```python
from build123d import *

# Parameters (mm, degrees)
F0_W     = 180
F0_H     = 150
F1_DEPTH = 20
F2_W     = 10
F2_H     = 150
F3_DEPTH = 20


# Not quite as in the source:
# - the program builds the solid bodies; features that only make, move or delete a surface that nothing else refers to are left out


with BuildPart() as f1:
    # F0 (on Right) → F1 (new body)
    with BuildSketch(Plane.YZ):
        with Locations((6.5838837624, 31.891247511)):
            Rectangle(F0_W, F0_H)
    extrude(amount=F1_DEPTH)

    # F2 (on face) → F3 (cut)
    with BuildSketch(Plane.XZ.offset(83.4161162376)):
        with Locations((15, 31.891247511)):
            Rectangle(F2_W, F2_H)
    extrude(amount=-F3_DEPTH, mode=Mode.SUBTRACT)


solid = f1.part
```
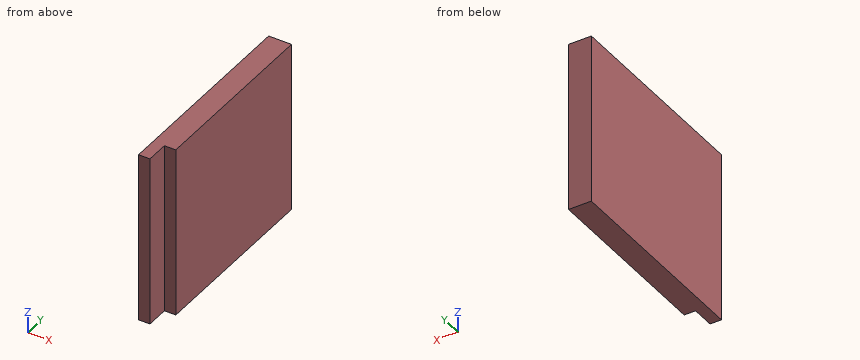
Geometry check sheet. Reference: the model listing, model coordinates, mm. Coordinates: 2 decimals unless noted, no trailing zeros. Loops run counter-clockwise (first coordinate to the right, second up) from the corner with the lowest first, then second, coordinate; pieces in that order, holes last.
Item 1: Sectioned sample at B-B, the plane x = 16. Record the boundary of the cut face in (y, z).
Item 2: Sectioned sample at A-A, the plane z = 19.5. Record the boundary of the cut face in (x, y), then the cut area to 3 significant figures.
Item 3: Go/stop test with a flat-tipped pin: pin 1 Ø6 at (y, z) = (-76, 4) entering from +X. Record where the tip stops, or that it passes through.
Item 4: Thickness scan on line 1 (Y direction, x = 18, z = 76). Record the ranges inside material, lowest first.
Check result:
1. outline: (-63.42, -43.11) - (96.58, -43.11) - (96.58, 106.89) - (-63.42, 106.89) - close
2. outline: (0, -83.42) - (10, -83.42) - (10, -63.42) - (20, -63.42) - (20, 96.58) - (0, 96.58) - close
2. area: 3,400 mm2
3. pin 1: stops at x = 10
4. line 1: y = -63.42 to 96.58
